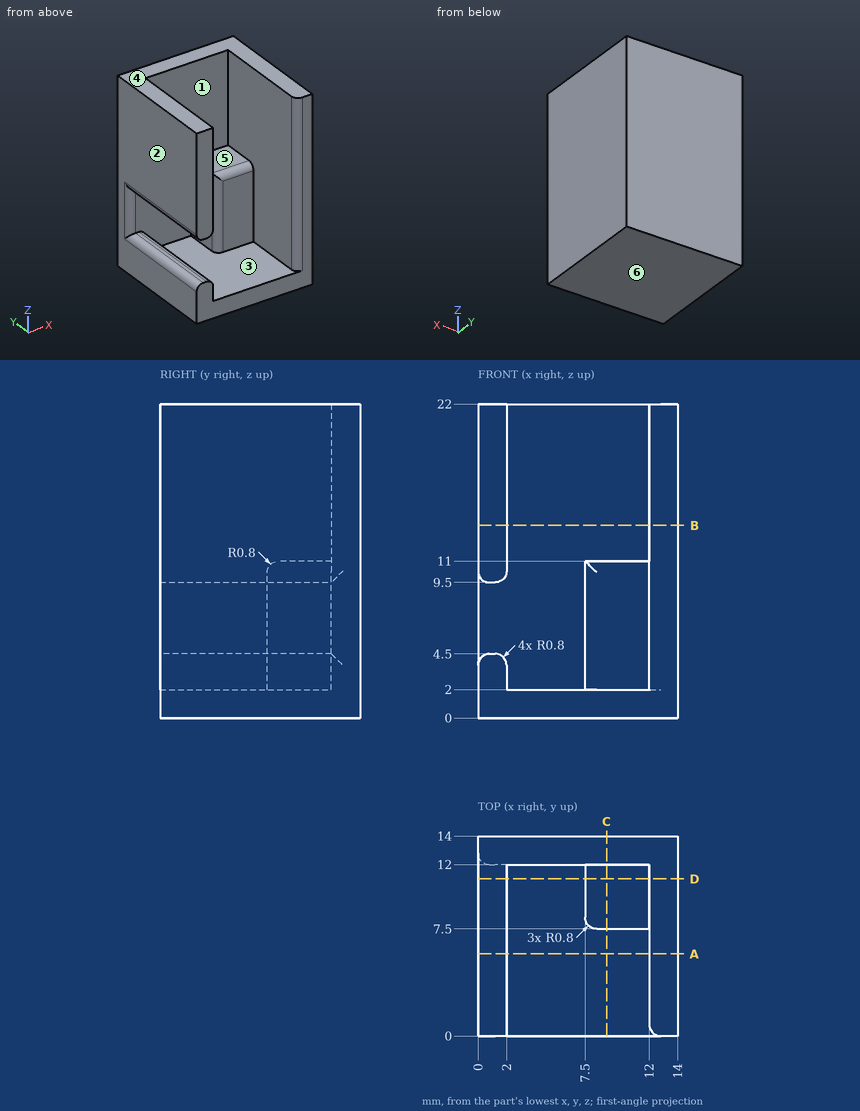
Could you check a few things on this drawing? It's one solid part, dimensions in mm from its lowest x, y, z. A direction names the side the tool comes from. Coordinates: 2 decimals unless noted, no trailing zeros. Order: outer loops, then holes, each group sorted by start corner. A loop starts at its lowest first (then second) coordinate and runs counter-clockwise, first axis right, second up. Notation, with made-up numbers: M 19.25,45 L 51.25,45 A27 cw 51.25,74 Z; hole C 59,73.25 d9. An arc over 180 degrees is marked long. Answer as a JSON object with one key per item and string values. Group by question number.
(1) Suppose I cut it at D-D, the plane y = 11. Please give me the cut outline in (x, z), then the cut area to 3 significant figures.
(2) I need wall thicknesses on probe 1 along X at (y, z) = (4, 11.75); probe 2 along Y at (x, z) = (1.75, 9.5); probe 3 along Z at (x, y) = (2.5, 1.5). Which ranges of each line are inside material? Lowest first, please.
(3) Suppose I cut it at C-C, the plane x = 9. Please give me the cut outline in (y, z), then the cut area to 3 significant figures.
(4) If we mould it in two halves opening along X, with no side actions, what happens to the marked faces 1, 2, 3 and 4? For each: released by +X, released by -X, zero draft, split by the parting line, or undercut.
(5) Suppose I cut it at B-B, the plane z = 13.5. Please give me the cut outline in (x, y), then the cut area to 3 significant figures.
(6) For pin 1 (3.5 mm diameter, centred on x = 6.5, z = 15, fed in from -Y); pin 2 (3 mm diameter, centred on y = 9, z = 6.5, fed in from -X); pin 3 (2 mm diameter, centred on x = 9.5, y = 5, fed in from +Z), each with a flat end and sliding along its axis, tell me the tip position at first contact or that it passes through.
(7) Which directions (+Z, -Z, +X, -X, +Y, -Y) give clear straight access to the entire face, cutting with the end or side of a thin tool? Please do the marked faces 5 and 6.
(8) Suppose I cut it at A-A, the plane y = 5.75. Please give me the cut outline in (x, z), then the cut area to 3 significant figures.
Values found:
{
 "1": {"outline": "M 0,0 L 14,0 L 14,22 L 12,22 L 12,11 L 7.5,11 L 7.5,2 L 2,2 L 2,3.7 A0.8 ccw 1.2,4.5 L 0.8,4.5 A0.8 ccw 0,3.7 Z; M 0,10.3 A0.8 ccw 0.8,9.5 L 1.2,9.5 A0.8 ccw 2,10.3 L 2,22 L 0,22 Z", "area": "138 mm^2"},
 "2": {"probe 1": "x = 0 to 2, 12 to 14", "probe 2": "y = 12 to 14", "probe 3": "z = 0 to 2"},
 "3": {"outline": "M 0,0 L 14,0 L 14,22 L 12,22 L 12,11 L 8.3,11 A0.8 ccw 7.5,10.2 L 7.5,2 L 0,2 Z", "area": "108 mm^2"},
 "4": {"face 1": "undercut", "face 2": "released by -X", "face 3": "undercut", "face 4": "zero draft"},
 "5": {"outline": "M 0,0 L 2,0 L 2,12 L 12,12 L 12,0.8 A0.8 ccw 12.8,0 L 14,0 L 14,14 L 0,14 Z", "area": "75.9 mm^2"},
 "6": {"pin 1": "stops at y = 12", "pin 2": "stops at x = 7.5", "pin 3": "stops at z = 2"},
 "7": {"face 5": "+Z, -Y", "face 6": "-Z, +X, -X, +Y, -Y"},
 "8": {"outline": "M 0,0 L 14,0 L 14,22 L 12,22 L 12,2 L 2,2 L 2,3.7 A0.8 ccw 1.2,4.5 L 0.8,4.5 A0.8 ccw 0,3.7 Z; M 0,10.3 A0.8 ccw 0.8,9.5 L 1.2,9.5 A0.8 ccw 2,10.3 L 2,22 L 0,22 Z", "area": "97.5 mm^2"}
}
